from build123d import *

# Parameters (mm, degrees)
FLANGE_BASE1_DEPTH             = 3
CORTE_EXTRUS_O1_DEPTH          = 3
ARESTA_FLANGE4_STRIP_W         = 13.4732
ARESTA_FLANGE4_STRIP_H         = 3
ARESTA_FLANGE4_STRIP_CUT_DEPTH = 18.4
ARESTA_FLANGE4_DEPTH           = 18.4
ESBO_O47_W                     = 14.5
ESBO_O47_H                     = 15
RESSALTO_EXTRUS_O1_DEPTH       = 3
FILETE1_R                      = 5
ESBO_O48_W                     = 14.5
ESBO_O48_H                     = 15
RESSALTO_EXTRUS_O2_DEPTH       = 3
FILETE2_R                      = 5
FILETE3_R                      = 2
CORTE_EXTRUS_O5_DEPTH          = 42.725642599
CORTE_EXTRUS_O6_DEPTH          = 3


# Sheet-metal steps are written as plain solids
with BuildPart() as part:
    # Esboço1 → Flange-base1 (new body)
    with BuildSketch(Plane.XY):
        Polygon((-14.370772566, 2.693459119), (-4.370772566, 2.693459119), (-4.370772566, 5.693459119), (14.029227434, 5.693459119), (14.029227434, 2.693459119), (21.029227434, 2.693459119), (21.029227434, -4.306540881), (-14.370772566, -4.306540881), align=None)
    extrude(amount=-FLANGE_BASE1_DEPTH)

    # Esboço8 → Corte-extrusão1 (cut)
    with BuildSketch(Plane.XY):
        with BuildLine():
            Line((-10.260200759, 1.193459119), (-2.260200759, 1.193459119))
            ThreePointArc((-2.260200759, 1.193459119), (-0.260200759, -0.806540881), (-2.260200759, -2.806540881))
            Line((-2.260200759, -2.806540881), (-10.260200759, -2.806540881))
            ThreePointArc((-10.260200759, -2.806540881), (-12.260200759, -0.806540881), (-10.260200759, 1.193459119))
        make_face()
        with BuildLine():
            Line((8.88097681, 1.193459119), (17.620096532, 1.193459119))
            ThreePointArc((17.620096532, 1.193459119), (19.620096532, -0.806540881), (17.620096532, -2.806540881))
            Line((17.620096532, -2.806540881), (8.88097681, -2.806540881))
            ThreePointArc((8.88097681, -2.806540881), (6.88097681, -0.806540881), (8.88097681, 1.193459119))
        make_face()
    extrude(amount=-CORTE_EXTRUS_O1_DEPTH, mode=Mode.SUBTRACT)

    # Aresta-Flange4 strip (across the edge) → Aresta-Flange4 strip cut (cut)
    with BuildSketch(Plane(origin=(14.029227434, 5.693459119, 0), x_dir=(0, -1, 0), z_dir=(-1, 0, 0))):
        with Locations((-6, -1.5)):
            Rectangle(ARESTA_FLANGE4_STRIP_W, ARESTA_FLANGE4_STRIP_H)
    extrude(amount=ARESTA_FLANGE4_STRIP_CUT_DEPTH, mode=Mode.SUBTRACT)

    # Aresta-Flange4 section (across the edge) → Aresta-Flange4 (add)
    with BuildSketch(Plane(origin=(14.029227434, 5.693459119, 0), x_dir=(0, -1, 0), z_dir=(-1, 0, 0))):
        with BuildLine():
            Line((-3, 0.7366), (-3, 22.5))
            Line((-3, 22.5), (0, 22.5))
            Line((0, 22.5), (0, 0.7366))
            ThreePointArc((0, 0.7366), (0.215745145, 0.215745145), (0.7366, 0))
            Line((0.7366, 0), (0.7366, -3))
            ThreePointArc((0.7366, -3), (-1.905575199, -1.905575199), (-3, 0.7366))
        make_face()
    extrude(amount=ARESTA_FLANGE4_DEPTH)

    # Esboço47 → Ressalto-extrusão1 (add)
    with BuildSketch(Plane(origin=(14.029227434, 0, 0), x_dir=(0, 0, -1), z_dir=(1, 0, 0))):
        with Locations((-15.25, 13.193459119)):
            Rectangle(ESBO_O47_W, ESBO_O47_H)
    extrude(amount=-RESSALTO_EXTRUS_O1_DEPTH)

    # Filete1
    filete1_edges = [part.edges().sort_by_distance(p)[0] for p in [
        (12.529227434, 20.693459119, 22.5),
        (12.529227434, 8.693459119, 8),
        (12.529227434, 20.693459119, 8),
    ]]
    fillet(filete1_edges, radius=FILETE1_R)

    # Esboço48 → Ressalto-extrusão2 (add)
    with BuildSketch(Plane.ZY.offset(4.370772566)):
        with Locations((15.25, 13.193459119)):
            Rectangle(ESBO_O48_W, ESBO_O48_H)
    extrude(amount=-RESSALTO_EXTRUS_O2_DEPTH)

    # Filete2
    filete2_edges = [part.edges().sort_by_distance(p)[0] for p in [
        (-2.870772566, 20.693459119, 22.5),
        (-2.870772566, 8.693459119, 8),
        (-2.870772566, 20.693459119, 8),
    ]]
    fillet(filete2_edges, radius=FILETE2_R)

    # Filete3
    filete3_edges = [part.edges().sort_by_distance(p)[0] for p in [
        (21.029227434, -4.306540881, -1.5),
        (-14.370772566, -4.306540881, -1.5),
        (-14.370772566, 2.693459119, -1.5),
        (-4.370772566, 2.693459119, -1.5),
        (14.029227434, 2.693459119, -1.5),
        (21.029227434, 2.693459119, -1.5),
    ]]
    fillet(filete3_edges, radius=FILETE3_R)

    # Esboço49 → Corte-extrusão5 (cut, through all)
    with BuildSketch(Plane(origin=(14.029227434, 0, 0), x_dir=(0, 0, -1), z_dir=(1, 0, 0))):
        with BuildLine():
            Line((-18.2, 11.175198381), (-12.3, 11.175198381))
            ThreePointArc((-12.3, 11.175198381), (-10.885786438, 11.760984819), (-10.3, 13.175198381))
            Line((-10.3, 13.175198381), (-10.3, 17.289297618))
            ThreePointArc((-10.3, 17.289297618), (-10.885786438, 18.70351118), (-12.3, 19.289297618))
            Line((-12.3, 19.289297618), (-18.2, 19.289297618))
            ThreePointArc((-18.2, 19.289297618), (-19.614213562, 18.70351118), (-20.2, 17.289297618))
            Line((-20.2, 17.289297618), (-20.2, 13.175198381))
            ThreePointArc((-20.2, 13.175198381), (-19.614213562, 11.760984819), (-18.2, 11.175198381))
        make_face()
    extrude(amount=-CORTE_EXTRUS_O5_DEPTH, mode=Mode.SUBTRACT)

    # Esboço50 → Corte-extrusão6 (cut)
    with BuildSketch(Plane.XZ.offset(-5.693459119)):
        with BuildLine():
            Line((1.629227434, 19.2366), (8.029227434, 19.2366))
            ThreePointArc((8.029227434, 19.2366), (9.443440996, 18.650813562), (10.029227434, 17.2366))
            Line((10.029227434, 17.2366), (10.029227434, 5.2366))
            ThreePointArc((10.029227434, 5.2366), (9.443440996, 3.822386438), (8.029227434, 3.2366))
            Line((8.029227434, 3.2366), (1.629227434, 3.2366))
            ThreePointArc((1.629227434, 3.2366), (0.215013871, 3.822386438), (-0.370772566, 5.2366))
            Line((-0.370772566, 5.2366), (-0.370772566, 17.2366))
            ThreePointArc((-0.370772566, 17.2366), (0.215013871, 18.650813562), (1.629227434, 19.2366))
        make_face()
    extrude(amount=-CORTE_EXTRUS_O6_DEPTH, mode=Mode.SUBTRACT)


solid = part.part
Could you check a few things on this model? Use its own coordinates, in mm. A direction names the side the tool comes from. Give positions to 0.01 mm unless a question says otherwise; leave off trailing zeros. Order: outer loops, then holes, each group sorted by start corner. A loop starts at its lowest first (then second) coordinate and runs counter-clockwise, first axis right, second up. Notation, with made-up numbers: (65.5, -40) -> (83.5, -40) arc R16 cw to (83.5, -29) -> close; hole circle Ø5 at (3, 8.5). An arc over 180 degrees is marked (long way). Return JSON: item names as keys, results as strings.
1. I need wall thicknesses on line 1 (Y direction, x = -1, z = 21.5); line 2 (X direction, y = 4.5, z = -0.5); line 3 (Z direction, x = -3.5, y = 2.25). Which ranges of each line are inside material? Lowest first, please. Write a range as from..to.
Answer list:
{"line 1": "y = 5.69..8.69", "line 2": "x = -4.38..14.04", "line 3": "z = -3..0"}
2. Imagine slicing it at C-C on x = 17. List the corners of the cut face in (y, z) for me.
Answer list:
{"outline": "(-4.31, -3) -> (-2.81, -3) -> (-2.81, 0) -> (-4.31, 0) -> close; (1.19, -3) -> (2.69, -3) -> (2.69, 0) -> (1.19, 0) -> close"}
3. Thinking about a two-plate mould opening in X: for faces 1 (the cylindrical face through (0.23, 7.17, 3.81)), 2 (the cylindrical face through (20.459, -3.705, -1.521)), 3 (the flat face through (-3, 15, 10.3)), which applies, pulls with the +X half, pulls with the -X half, needs draft (parallel to the pull), parting line crosses it, or undercut?
Answer list:
{"face 1": "undercut", "face 2": "pulls with the +X half", "face 3": "needs draft"}
4. On a 3-axis mill with a long thin cutter (end or side, diameter ignored), from which of +Z, -Z, +X, -X, +Y, -Y can I reach the whole of each face in a straight line? I mean faces 4 (the flat face through (11.029, 11, 15)), 5 (the cylindrical face through (6.88, -0.85, -1.48)), 6 (the flat face through (-3, 15, 8)), 7 (the cylindrical face through (9.46, 7.17, 3.84)). Say none if no direction works.
Answer list:
{"face 4": "+Z, -Z, +Y", "face 5": "+Z, -Z", "face 6": "-Z, +X, -X, +Y", "face 7": "+Y, -Y"}
5. Imagine slicing it at D-D on y = 10.5. List the corners of the cut face in (x, z) for me, then the cut area to 3 significant figures.
Answer list:
{"outline": "(-4.37, 6.85) -> (-1.37, 6.85) -> (-1.37, 22.5) -> (-4.37, 22.5) -> close; (11.03, 6.85) -> (14.03, 6.85) -> (14.03, 22.5) -> (11.03, 22.5) -> close", "area": "93.9 mm2"}
6. Imagine slicing it at B-B on z = 14. List the corners of the cut face in (x, y) for me.
Answer list:
{"outline": "(-4.37, 5.69) -> (-0.37, 5.69) -> (-0.37, 8.69) -> (-1.37, 8.69) -> (-1.37, 11.18) -> (-4.37, 11.18) -> close; (-4.37, 19.29) -> (-1.37, 19.29) -> (-1.37, 20.69) -> (-4.37, 20.69) -> close; (10.03, 5.69) -> (14.03, 5.69) -> (14.03, 11.18) -> (11.03, 11.18) -> (11.03, 8.69) -> (10.03, 8.69) -> close; (11.03, 19.29) -> (14.03, 19.29) -> (14.03, 20.69) -> (11.03, 20.69) -> close"}
7. Imagine slicing it at A-A on x = 11.5. List the corners of the cut face in (y, z) for me.
Answer list:
{"outline": "(-4.31, -3) -> (-2.81, -3) -> (-2.81, 0) -> (-4.31, 0) -> close; (1.19, -3) -> (4.96, -3) arc R3.74 ccw to (8.69, 0.74) -> (8.69, 3) arc R5 cw to (13.69, 8) -> (15.69, 8) arc R5 ccw to (20.69, 13) -> (20.69, 17.5) arc R5 ccw to (15.69, 22.5) -> (5.69, 22.5) -> (5.69, 0.74) arc R0.74 cw to (4.96, 0) -> (1.19, 0) -> close; hole (11.18, 12.3) arc R2 ccw to (13.18, 10.3) -> (17.29, 10.3) arc R2 ccw to (19.29, 12.3) -> (19.29, 18.2) arc R2 ccw to (17.29, 20.2) -> (13.18, 20.2) arc R2 ccw to (11.18, 18.2) -> close"}
8. For pin 1 Ø1.5 at (x, z) = (18, -2) entering from +Y; pin 2 Ø8 at (x, z) = (15, 10.5) entering from -Y; pin 3 Ø1.6 at (x, y) = (-3, 14.5) entering from -Z; pin 4 Ø5 at (x, y) = (14.5, 16.5) entering from +Z, each with a flat end and sliding along its axis, tell me the tip position at first contact or that it passes through.
Answer list:
{"pin 1": "stops at y = 2.69", "pin 2": "stops at y = 5.69", "pin 3": "stops at z = 8", "pin 4": "stops at z = 22.5"}
